Answer from the drawing. Dimensions are ordinates in mm from the lowest x, y and z of the part. Give positions to 0.01 mm unless a question says otherwise; leave off trailing zeros. Order: outer loops, then holes, each group sorted by start corner. A loop starts at its lowest first (then second) coordinate and runs counter-clockwise, first axis right, second up. Notation, with made-up numbers: (41, 36) -> (49, 36) arc R18 ccw to (49, 49) -> close; hole circle Ø7 at (-4, 64). An arc over 180 degrees is marked (long way). Answer as a JSON object with one key per item and string values. Group by question number.
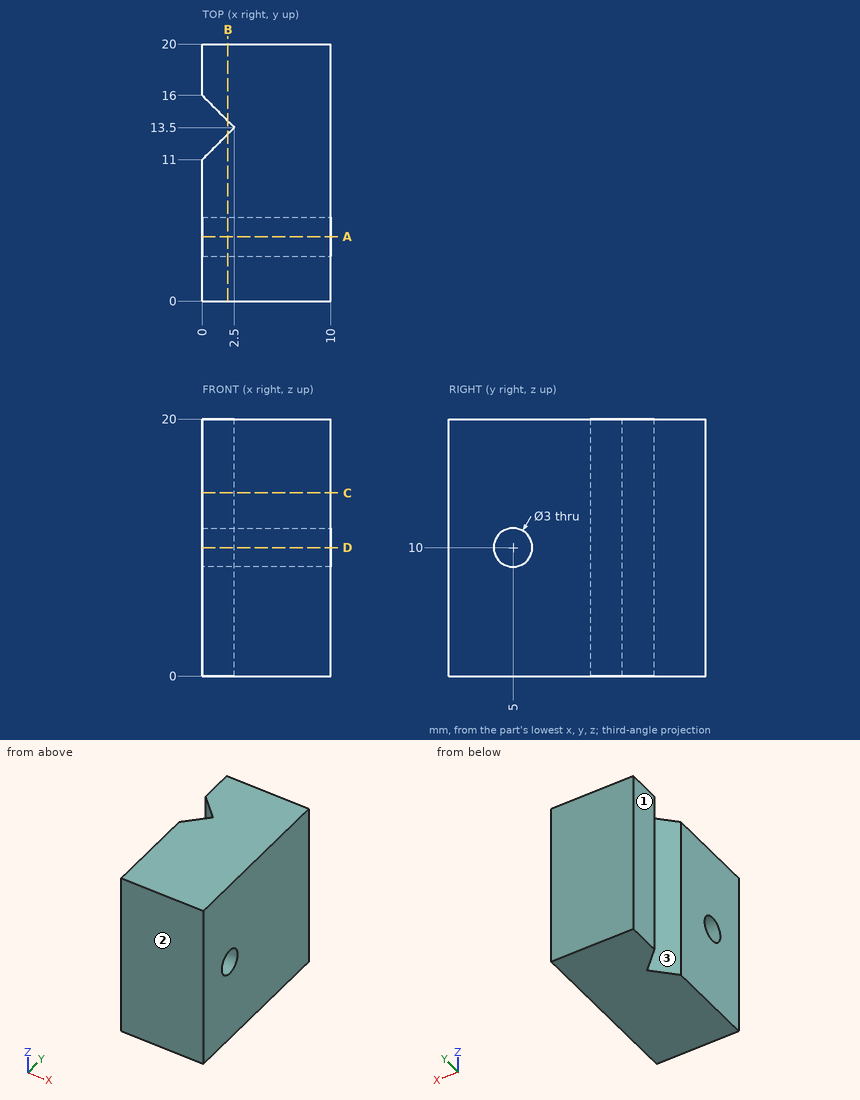
(1) A flat-ended cylindrical pin translates along its axis: pin 1 Ø4 at (y, z) = (12.5, 2.5) entering from -X. Find the tip coordinate at first contact, or state that the pin passes through.
(2) A cutting plane is placed at C-C (z = 14.25). Determine the outline of the cut face in (x, y), and give its area (3 significant figures).
(3) A cutting plane is placed at B-B (x = 2). Determine the outline of the cut face in (y, z), and give its area (3 significant figures).
(4) A cutting plane is placed at A-A (y = 5). Determine the outline of the cut face in (x, z).
(5) For a pull along Y with two mould halves and no side action, classify the marked faces 1, 2 and 3 as +Y half, -Y half, draft (parallel to the pull), parting line (faces both ways), or undercut.
(6) Find the intervals of material crossed by line 1 along Y through (x, z) = (2.25, 10); line 2 along Y through (x, z) = (5.5, 10); line 3 along Y through (x, z) = (3.75, 8.75), in increasing order. Write a range as [from, to].
(7) A cutting plane is placed at D-D (z = 10). Determine the outline of the cut face in (x, y), and give its area (3 significant figures).
Check sheet entries:
{
 "1": {"pin 1": "stops at x = 0"},
 "2": {"outline": "(0, 0) -> (10, 0) -> (10, 20) -> (0, 20) -> (0, 16) -> (2.5, 13.5) -> (0, 11) -> close", "area": "194 mm2"},
 "3": {"outline": "(0, 0) -> (13, 0) -> (13, 20) -> (0, 20) -> close; (14, 0) -> (20, 0) -> (20, 20) -> (14, 20) -> close; hole circle Ø3 at (5, 10)", "area": "373 mm2"},
 "4": {"outline": "(0, 0) -> (10, 0) -> (10, 8.5) -> (0, 8.5) -> close; (0, 11.5) -> (10, 11.5) -> (10, 20) -> (0, 20) -> close"},
 "5": {"face 1": "draft", "face 2": "-Y half", "face 3": "undercut"},
 "6": {"line 1": "y = [0, 3.5], [6.5, 13.25], [13.75, 20]", "line 2": "y = [0, 3.5], [6.5, 20]", "line 3": "y = [0, 4.17], [5.83, 20]"},
 "7": {"outline": "(0, 0) -> (10, 0) -> (10, 3.5) -> (0, 3.5) -> close; (0, 6.5) -> (10, 6.5) -> (10, 20) -> (0, 20) -> (0, 16) -> (2.5, 13.5) -> (0, 11) -> close", "area": "164 mm2"}
}
